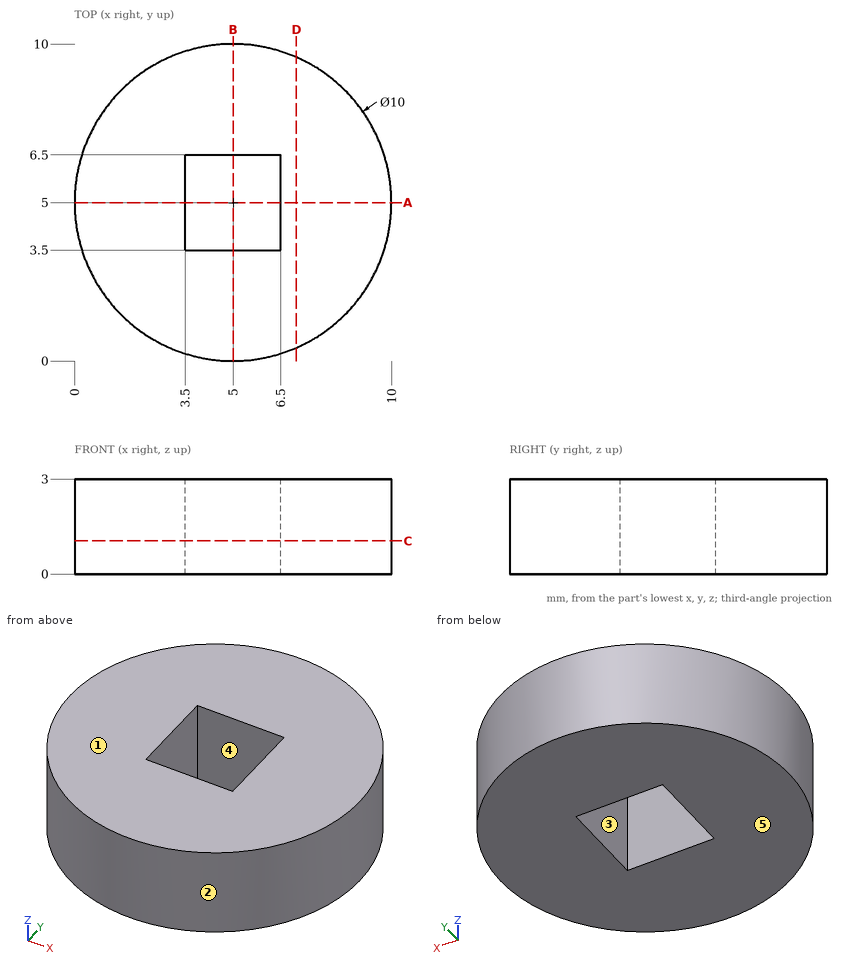
Job drawing, mm, ordinate dimensions from the low corner. One solid piece. A direction names the side the tool comes from. Coordinates: 2 decimals unless noted, no trailing zeros. Loops run counter-clockwise (first coordinate to the right, second up) from the corner with the lowest first, then second, coordinate; pieces in that order, holes last. Notation, with made-up numbers: (62, 38.25) -> (121, 38.25) arc R34 cw to (121, 77.25) -> close; hole circle Ø9 at (-15.5, 74.5). An arc over 180 degrees is marked (long way). One line per item, written item: value.
1. Drill centre lines: line 1 (X direction, y = 4.25, z = 0.65); line 2 (Y direction, x = 4, z = 0.2); line 3 (X direction, y = 5.5, z = 2.2). Where is each one in solid material? Low to high. Write a range as [from, to].
Answers:
line 1: x = [0.06, 3.5], [6.5, 9.94]
line 2: y = [0.1, 3.5], [6.5, 9.9]
line 3: x = [0.03, 3.5], [6.5, 9.97]
2. Flat gauge pin, fed straight in: P1, Ø1, axis at y = 8, z = 2, coming from the +X side. Where does the tip first touch, or does it go through?
Answers:
P1: stops at x = 9.33
3. Which spindle directions (+Z, -Z, +X, -X, +Y, -Y) get a long thin tool onto all of the face, cutting with end or side? Do the marked faces 4 and 5. Say none if no direction does.
Answers:
face 4: +Z, -Z
face 5: -Z, +X, -X, +Y, -Y
4. Slice it at C-C on z = 1.05. Write the cut outline in (x, y).
Answers:
outline: circle Ø10 at (5, 5); hole (3.5, 3.5) -> (6.5, 3.5) -> (6.5, 6.5) -> (3.5, 6.5) -> close
5. Pull direction X, two halves, no side cores. Call the marked faces 1, 2 and 3: pulls with the +X half, pulls with the -X half, needs draft (parallel to the pull), parting line crosses it, or undercut.
Answers:
face 1: needs draft
face 2: parting line crosses it
face 3: undercut
6. Slice it at D-D on x = 7. Write the cut outline in (y, z), and give its area (3 significant figures).
Answers:
outline: (0.42, 0) -> (9.58, 0) -> (9.58, 3) -> (0.42, 3) -> close
area: 27.5 mm^2
7. Slice it at A-A on y = 5. Write the cut outline in (x, z).
Answers:
outline: (0, 0) -> (3.5, 0) -> (3.5, 3) -> (0, 3) -> close; (6.5, 0) -> (10, 0) -> (10, 3) -> (6.5, 3) -> close
